Geometry check sheet. Reference: the model listing, model coordinates, mm. A direction names the side the tool comes from. Round coordinates to 2 decimals unless told otherwise and drop trailing zeros. Order: outer loops, then holes, each group sorted by start corner. A loop starts at its lowest first (then second) coordinate and runs counter-clockwise, first axis right, second up.
```python
from build123d import *

# Parameters (mm, degrees)
SKIZZE1_W                                 = 98
SKIZZE1_H                                 = 50
SKIZZE1_W_2                               = 102
SKIZZE1_H_2                               = 57.5
AUFSATZ_LINEAR_AUSTRAGEN1_DEPTH           = 15
SKIZZE4_W                                 = 98
SKIZZE4_H                                 = 50
SCHNITT_LINEAR_AUSTRAGEN1_DEPTH           = 13.5
SKIZZE5_R                                 = 3.25
AUFSATZ_LINEAR_AUSTRAGEN2_DEPTH           = 1.5
SCHNITT_LINEAR_AUSTRAGEN3_REACH           = 120.048
SCHNITT_LINEAR_AUSTRAGEN4_REACH           = 120.048
AUFSATZ_LINEAR_AUSTRAGEN3_DEPTH           = 1.5
M3_GEWINDEBOHRUNG1_D                      = 2.5
GEWINDEBOHRUNG_F_R_M4X0_7_HELICOIL1_D     = 4.2
GEWINDEBOHRUNG_F_R_M4X0_7_HELICOIL1_DEPTH = 4
GEWINDEBOHRUNG_F_R_M4X0_7_HELICOIL1_TIP   = 1.2618073
VERRUNDUNG1_R                             = 5
VERRUNDUNG2_R                             = 3
VERRUNDUNG3_R                             = 1
VERRUNDUNG4_R                             = 3
M2_GEWINDEBOHRUNG1_D                      = 1.6
M2_GEWINDEBOHRUNG1_DEPTH                  = 6
M2_GEWINDEBOHRUNG1_TIP                    = 0.480688495
SCHNITT_LINEAR_AUSTRAGEN5_DEPTH           = 119.047659867
SKIZZE20_R                                = 2.25
AUFSATZ_LINEAR_AUSTRAGEN4_DEPTH           = 3
VERRUNDUNG5_R                             = 3
SKIZZE21_R                                = 2.25
SKIZZE21_W                                = 52
SKIZZE21_H                                = 6
SKIZZE21_W_2                              = 16
SKIZZE21_H_2                              = 16.5
SKIZZE21_W_3                              = 6
SKIZZE21_H_3                              = 10
SCHNITT_LINEAR_AUSTRAGEN6_DEPTH           = 0.75
VERRUNDUNG6_R                             = 3


with BuildPart() as part:
    # Skizze1 → Aufsatz-Linear austragen1 (new body)
    with BuildSketch(Plane.XY):
        with Locations((51, 26.5)):
            Rectangle(SKIZZE1_W, SKIZZE1_H)
        with Locations((51, 28.75)):
            Rectangle(SKIZZE1_W_2, SKIZZE1_H_2)
    extrude(amount=AUFSATZ_LINEAR_AUSTRAGEN1_DEPTH)

    # Skizze4 → Schnitt-Linear austragen1 (cut)
    with BuildSketch(Plane.XY.offset(15)):
        with Locations((51, 26.5)):
            Rectangle(SKIZZE4_W, SKIZZE4_H)
    extrude(amount=-SCHNITT_LINEAR_AUSTRAGEN1_DEPTH, mode=Mode.SUBTRACT)

    # Skizze5 → Aufsatz-Linear austragen2 (add)
    with BuildSketch(Plane.XY.offset(1.5)):
        with Locations((6.235, 5.55)):
            Circle(SKIZZE5_R)
        with Locations((55.765, 5.55)):
            Circle(SKIZZE5_R)
        with Locations((95.765, 5.55)):
            Circle(SKIZZE5_R)
        with Locations((95.765, 47.45)):
            Circle(SKIZZE5_R)
        with Locations((6.235, 47.45)):
            Circle(SKIZZE5_R)
    extrude(amount=AUFSATZ_LINEAR_AUSTRAGEN2_DEPTH)

    # Skizze11 → Schnitt-Linear austragen3 (cut, up to next)
    with BuildSketch(Plane.ZY, mode=Mode.PRIVATE) as schnitt_linear_austragen3_sk1:
        with BuildLine():
            Line((17, 37.75), (17, 22.75))
            ThreePointArc((17, 22.75), (9.5, 30.25), (17, 37.75))
        make_face()
    schnitt_linear_austragen3_tool1 = extrude(schnitt_linear_austragen3_sk1.sketch, amount=-SCHNITT_LINEAR_AUSTRAGEN3_REACH, mode=Mode.PRIVATE) & part.part
    add(schnitt_linear_austragen3_tool1.solids().sort_by_distance((0, 30.25, 13.816901))[0], mode=Mode.SUBTRACT)

    # Skizze12 → Schnitt-Linear austragen4 (cut, up to next)
    with BuildSketch(Plane(origin=(0, 57.5, 0), x_dir=(1, 0, 0), z_dir=(0, 1, 0)), mode=Mode.PRIVATE) as schnitt_linear_austragen4_sk1:
        with BuildLine():
            Line((85, -5.75), (85, -15))
            Line((85, -15), (31, -15))
            Line((31, -15), (31, -5.75))
            ThreePointArc((31, -5.75), (31.439339828, -4.689339828), (32.5, -4.25))
            Line((32.5, -4.25), (83.5, -4.25))
            ThreePointArc((83.5, -4.25), (84.560660172, -4.689339828), (85, -5.75))
        make_face()
    schnitt_linear_austragen4_tool1 = extrude(schnitt_linear_austragen4_sk1.sketch, amount=-SCHNITT_LINEAR_AUSTRAGEN4_REACH, mode=Mode.PRIVATE) & part.part
    add(schnitt_linear_austragen4_tool1.solids().sort_by_distance((58, 57.5, 9.633398))[0], mode=Mode.SUBTRACT)

    # Skizze13 → Aufsatz-Linear austragen3 (add)
    with BuildSketch(Plane.XY.offset(1.5)):
        with BuildLine():
            Line((6.235, 44.2), (2, 44.2))
            Line((2, 44.2), (2, 51.5))
            Line((2, 51.5), (9.485, 51.5))
            Line((9.485, 51.5), (9.485, 47.45))
            ThreePointArc((9.485, 47.45), (8.533097039, 45.151902961), (6.235, 44.2))
        make_face()
        with BuildLine():
            Line((9.485, 5.55), (9.485, 1.5))
            Line((9.485, 1.5), (2, 1.5))
            Line((2, 1.5), (2, 8.8))
            Line((2, 8.8), (6.235, 8.8))
            ThreePointArc((6.235, 8.8), (8.533097039, 7.848097039), (9.485, 5.55))
        make_face()
        with BuildLine():
            Line((100, 1.5), (100, 8.8))
            Line((100, 8.8), (95.765, 8.8))
            ThreePointArc((95.765, 8.8), (93.466902961, 7.848097039), (92.515, 5.55))
            Line((92.515, 5.55), (92.515, 1.5))
            Line((92.515, 1.5), (100, 1.5))
        make_face()
        with BuildLine():
            Line((100, 51.5), (92.515, 51.5))
            Line((92.515, 51.5), (92.515, 47.45))
            ThreePointArc((92.515, 47.45), (93.466902961, 45.151902961), (95.765, 44.2))
            Line((95.765, 44.2), (100, 44.2))
            Line((100, 44.2), (100, 51.5))
        make_face()
        with BuildLine():
            Line((59.015, 5.55), (59.015, 1.5))
            Line((59.015, 1.5), (52.515, 1.5))
            Line((52.515, 1.5), (52.515, 5.55))
            ThreePointArc((52.515, 5.55), (55.765, 8.8), (59.015, 5.55))
        make_face()
    extrude(amount=AUFSATZ_LINEAR_AUSTRAGEN3_DEPTH)

    # M3 Gewindebohrung1 (through all)
    with Locations(Plane.XY.offset(3)):
        with Locations((6.235, 47.45), (6.235, 5.55), (55.765, 5.55), (95.765, 47.45), (95.765, 5.55)):
            Hole(M3_GEWINDEBOHRUNG1_D / 2)

    # Gewindebohrung für M4x0.7 Helicoil1
    with Locations(Plane(origin=(38.515151917, 57.5, 4.646014508), x_dir=(-1, 0, 0), z_dir=(0, 1, 0))):
        with Locations((34.515151917, -0.646014508), (-59.484848083, -0.646014508)):
            Hole(GEWINDEBOHRUNG_F_R_M4X0_7_HELICOIL1_D / 2, depth=GEWINDEBOHRUNG_F_R_M4X0_7_HELICOIL1_DEPTH)
            with Locations((0, 0, -(GEWINDEBOHRUNG_F_R_M4X0_7_HELICOIL1_DEPTH + GEWINDEBOHRUNG_F_R_M4X0_7_HELICOIL1_TIP / 2))):  # 118° drill point
                Cone(0, GEWINDEBOHRUNG_F_R_M4X0_7_HELICOIL1_D / 2, GEWINDEBOHRUNG_F_R_M4X0_7_HELICOIL1_TIP, mode=Mode.SUBTRACT)

    # Verrundung1
    verrundung1_edges = [part.edges().sort_by_distance(p)[0] for p in [
        (2, 1.5, 9),
        (100, 1.5, 9),
    ]]
    fillet(verrundung1_edges, radius=VERRUNDUNG1_R)

    # Verrundung2
    verrundung2_edges = [part.edges().sort_by_distance(p)[0] for p in [
        (100, 44.2, 2.25),
        (92.515, 51.5, 2.25),
        (9.485, 51.5, 2.25),
        (2, 44.2, 2.25),
        (52.515, 1.5, 2.25),
        (59.015, 1.5, 2.25),
        (9.485, 1.5, 2.25),
        (2, 8.8, 2.25),
        (92.515, 1.5, 2.25),
        (100, 8.8, 2.25),
    ]]
    fillet(verrundung2_edges, radius=VERRUNDUNG2_R)

    # Verrundung3
    verrundung3_edges = [part.edges().sort_by_distance(p)[0] for p in [
        (0, 0, 7.5),
        (0, 57.5, 7.5),
        (102, 57.5, 7.5),
        (102, 0, 7.5),
    ]]
    fillet(verrundung3_edges, radius=VERRUNDUNG3_R)

    # Verrundung4
    verrundung4_edges = [part.edges().sort_by_distance(p)[0] for p in [
        (100, 51.5, 9),
        (2, 51.5, 9),
    ]]
    fillet(verrundung4_edges, radius=VERRUNDUNG4_R)

    # M2 Gewindebohrung1
    with Locations(Plane.XY.offset(15)):
        with Locations((1.9, 55.6), (100.1, 55.6), (100.1, 1.9), (1.9, 1.9)):
            Hole(M2_GEWINDEBOHRUNG1_D / 2, depth=M2_GEWINDEBOHRUNG1_DEPTH)
            with Locations((0, 0, -(M2_GEWINDEBOHRUNG1_DEPTH + M2_GEWINDEBOHRUNG1_TIP / 2))):  # 118° drill point
                Cone(0, M2_GEWINDEBOHRUNG1_D / 2, M2_GEWINDEBOHRUNG1_TIP, mode=Mode.SUBTRACT)

    # Skizze19 → Schnitt-Linear austragen5 (cut, through all)
    with BuildSketch(Plane.XY.offset(15)):
        with BuildLine():
            Line((94, 57.5), (8, 57.5))
            ThreePointArc((8, 57.5), (10.371708245, 56.901704215), (12.175823272, 55.25))
            ThreePointArc((12.175823272, 55.25), (13.979938299, 53.598295785), (16.351646544, 53))
            Line((16.351646544, 53), (85.648353456, 53))
            ThreePointArc((85.648353456, 53), (88.020061701, 53.598295785), (89.824176728, 55.25))
            ThreePointArc((89.824176728, 55.25), (91.628291755, 56.901704215), (94, 57.5))
        make_face()
    extrude(amount=-SCHNITT_LINEAR_AUSTRAGEN5_DEPTH, mode=Mode.SUBTRACT)

    # Skizze20 → Aufsatz-Linear austragen4 (add)
    with BuildSketch(Plane(origin=(0, 0, 0), x_dir=(-1, 0, 0), z_dir=(0, 0, -1))):
        Polygon((-47, -8), (-51, -8), (-55, -8), (-55, 0), (-47, 0), align=None)
        with Locations((-51, -4)):
            Circle(SKIZZE20_R, mode=Mode.SUBTRACT)
    extrude(amount=-AUFSATZ_LINEAR_AUSTRAGEN4_DEPTH)

    # Verrundung5
    verrundung5_edges = [part.edges().sort_by_distance(p)[0] for p in [
        (55, -8, 1.5),
        (55, 0, 1.5),
        (47, 0, 1.5),
        (47, -8, 1.5),
    ]]
    fillet(verrundung5_edges, radius=VERRUNDUNG5_R)

    # Skizze21 → Schnitt-Linear austragen6 (cut)
    with BuildSketch(Plane.XY.offset(1.5)):
        with Locations((89.465, 7.6)):
            Circle(SKIZZE21_R)
        with Locations((27.865, 7.6)):
            Circle(SKIZZE21_R)
        with Locations((57.765, 46.2)):
            Rectangle(SKIZZE21_W, SKIZZE21_H)
        with Locations((11.055, 30.2)):
            Rectangle(SKIZZE21_W_2, SKIZZE21_H_2)
        with Locations((97, 35.71)):
            Rectangle(SKIZZE21_W_3, SKIZZE21_H_3)
    extrude(amount=-SCHNITT_LINEAR_AUSTRAGEN6_DEPTH, mode=Mode.SUBTRACT)

    # Verrundung6
    verrundung6_edges = [part.edges().sort_by_distance(p)[0] for p in [
        (3.055, 21.95, 1.125),
        (3.055, 38.45, 1.125),
        (19.055, 38.45, 1.125),
        (19.055, 21.95, 1.125),
        (31.765, 43.2, 1.125),
        (31.765, 49.2, 1.125),
        (83.765, 49.2, 1.125),
        (83.765, 43.2, 1.125),
        (100, 30.71, 1.125),
        (94, 30.71, 1.125),
        (94, 40.71, 1.125),
        (100, 40.71, 1.125),
    ]]
    fillet(verrundung6_edges, radius=VERRUNDUNG6_R - 0.0001)  # a hair under: the kernel refuses the full size


solid = part.part
```
(1) Depth check by flat-ended pin: P1, Ø8, axis at x = 10.5, y = 34.5, coming from the +Z side; P2, Ø1.5, axis at x = 13, z = 4, coming from the -Y side; P3, Ø3, axis at x = 87, z = 3.5, coming from the +Y side. Enter the tip coordinate at first touch or a pass-through.
Returned:
P1: stops at z = 1.5
P2: stops at y = 0
P3: stops at y = 53.89
(2) Set-up check for faces 5 (the cylindrical face through (55.9, -0.86, 1.52)), 6 (the flat face through (100, 27, 8)): record each of +Z, -Z, +X, -X, +Y, -Y from which the full face is reachable in a straight line by a thin tool's end or side.
Returned:
face 5: +Z, -Z, +X, -Y
face 6: +Z
(3) Material ranges on line 1 (Y direction, x = 100.1, z = 10.9); line 2 (Z direction, x = 4, y = 56); line 3 (Y direction, x = 29, z = 11.5), recorded low to high.
Returned:
line 1: y = 0 to 1.1, 2.7 to 54.8, 56.4 to 57.5
line 2: z = 0 to 1.9, 6.1 to 15
line 3: y = 0 to 1.5, 51.5 to 53
(4) Sectioned sample at A-A, the plane x = 51. Record the cut outline in (y, z), and give its area (3 significant figures).
Returned:
outline: (-8, 0) - (-6.25, 0) - (-6.25, 3) - (-8, 3) - close; (-1.75, 0) - (53, 0) - (53, 4.25) - (51.5, 4.25) - (51.5, 1.5) - (49.2, 1.5) - (49.2, 0.75) - (43.2, 0.75) - (43.2, 1.5) - (1.89, 1.5) - (1.89, 3) - (1.5, 3) - (1.5, 15) - (0, 15) - (0, 3) - (-1.75, 3) - close
area: 110 mm2
(5) Draft check along X on faces 1 (the flat face through (50, 25, 0)), 2 (the cylindrical face through (99.14, 9.7, 2.26)), 3 (the cylindrical face through (54.14, -7.1, 1.52)), 4 (the cylindrical face through (46.1, -0.86, 1.52)). Enter one of: released by +X, released by -X, zero draft, split by the parting line, or undercut.
Returned:
face 1: zero draft
face 2: undercut
face 3: released by +X
face 4: released by -X
